from build123d import *

# Parameters (mm, degrees)
SKETCH3_W           = 186.436
SKETCH3_H           = 186.436
BOSS_EXTRUDE1_DEPTH = 3.0988
CUT_EXTRUDE1_DEPTH  = 264.678529186
CUT_EXTRUDE2_REACH  = 265.679
SKETCH5_R           = 3.175
SKETCH5_W           = 63.5
SKETCH5_H           = 63.5


with BuildPart() as part:
    # Sketch3 → Boss-Extrude1 (new body)
    with BuildSketch(Plane(origin=(0, 0, 0), x_dir=(1, 0, 0), z_dir=(0, 1, 0))):
        with Locations((93.218, 93.218)):
            Rectangle(SKETCH3_W, SKETCH3_H)
    extrude(amount=BOSS_EXTRUDE1_DEPTH)

    # Sketch4 → Cut-Extrude1 (cut, through all)
    with BuildSketch(Plane(origin=(0, 3.0988, 0), x_dir=(1, 0, 0), z_dir=(0, 1, 0))):
        with BuildLine():
            Line((5.842, 82.296), (29.718, 82.296))
            ThreePointArc((29.718, 82.296), (31.242, 80.772), (29.718, 79.248))
            Line((29.718, 79.248), (5.842, 79.248))
            ThreePointArc((5.842, 79.248), (4.318, 80.772), (5.842, 82.296))
        make_face()
        with BuildLine():
            Line((5.842, 104.14), (29.718, 104.14))
            ThreePointArc((29.718, 104.14), (31.242, 105.664), (29.718, 107.188))
            Line((29.718, 107.188), (5.842, 107.188))
            ThreePointArc((5.842, 107.188), (4.318, 105.664), (5.842, 104.14))
        make_face()
        with BuildLine():
            Line((80.772, 29.718), (80.772, 5.842))
            ThreePointArc((80.772, 5.842), (82.296, 4.318), (83.82, 5.842))
            Line((83.82, 5.842), (83.82, 29.718))
            ThreePointArc((83.82, 29.718), (82.296, 31.242), (80.772, 29.718))
        make_face()
        with BuildLine():
            Line((105.664, 5.842), (105.664, 29.718))
            ThreePointArc((105.664, 29.718), (104.14, 31.242), (102.616, 29.718))
            Line((102.616, 29.718), (102.616, 5.842))
            ThreePointArc((102.616, 5.842), (104.14, 4.318), (105.664, 5.842))
        make_face()
        with BuildLine():
            Line((156.718, 83.82), (180.594, 83.82))
            ThreePointArc((180.594, 83.82), (182.118, 82.296), (180.594, 80.772))
            Line((180.594, 80.772), (156.718, 80.772))
            ThreePointArc((156.718, 80.772), (155.194, 82.296), (156.718, 83.82))
        make_face()
        with BuildLine():
            Line((156.718, 102.616), (180.594, 102.616))
            ThreePointArc((180.594, 102.616), (182.118, 104.14), (180.594, 105.664))
            Line((180.594, 105.664), (156.718, 105.664))
            ThreePointArc((156.718, 105.664), (155.194, 104.14), (156.718, 102.616))
        make_face()
        with BuildLine():
            Line((80.772, 180.594), (80.772, 156.718))
            ThreePointArc((80.772, 156.718), (82.296, 155.194), (83.82, 156.718))
            Line((83.82, 156.718), (83.82, 180.594))
            ThreePointArc((83.82, 180.594), (82.296, 182.118), (80.772, 180.594))
        make_face()
        with BuildLine():
            Line((105.664, 156.718), (105.664, 180.594))
            ThreePointArc((105.664, 180.594), (104.14, 182.118), (102.616, 180.594))
            Line((102.616, 180.594), (102.616, 156.718))
            ThreePointArc((102.616, 156.718), (104.14, 155.194), (105.664, 156.718))
        make_face()
    extrude(amount=-CUT_EXTRUDE1_DEPTH, mode=Mode.SUBTRACT)

    # Sketch5 → Cut-Extrude2 (cut, up to next)
    with BuildSketch(Plane(origin=(0, 3.0988, 0), x_dir=(1, 0, 0), z_dir=(0, 1, 0)), mode=Mode.PRIVATE) as cut_extrude2_sk1:
        with Locations(Location((50.8, 63.5, 0), (0, 0, 270))):
            Circle(SKETCH5_R)
    cut_extrude2_tool1 = extrude(cut_extrude2_sk1.sketch, amount=-CUT_EXTRUDE2_REACH, mode=Mode.PRIVATE) & part.part
    # Sketch5 → Cut-Extrude2 (cut, up to next)
    with BuildSketch(Plane(origin=(0, 3.0988, 0), x_dir=(1, 0, 0), z_dir=(0, 1, 0)), mode=Mode.PRIVATE) as cut_extrude2_sk2:
        with Locations(Location((93.218, 63.5, 0), (0, 0, 270))):
            Circle(SKETCH5_R)
    cut_extrude2_tool2 = extrude(cut_extrude2_sk2.sketch, amount=-CUT_EXTRUDE2_REACH, mode=Mode.PRIVATE) & part.part
    # Sketch5 → Cut-Extrude2 (cut, up to next)
    with BuildSketch(Plane(origin=(0, 3.0988, 0), x_dir=(1, 0, 0), z_dir=(0, 1, 0)), mode=Mode.PRIVATE) as cut_extrude2_sk3:
        with Locations(Location((135.636, 63.5, 0), (0, 0, 270))):
            Circle(SKETCH5_R)
    cut_extrude2_tool3 = extrude(cut_extrude2_sk3.sketch, amount=-CUT_EXTRUDE2_REACH, mode=Mode.PRIVATE) & part.part
    # Sketch5 → Cut-Extrude2 (cut, up to next)
    with BuildSketch(Plane(origin=(0, 3.0988, 0), x_dir=(1, 0, 0), z_dir=(0, 1, 0)), mode=Mode.PRIVATE) as cut_extrude2_sk4:
        with Locations((93.218, 116.586)):
            Rectangle(SKETCH5_W, SKETCH5_H)
    cut_extrude2_tool4 = extrude(cut_extrude2_sk4.sketch, amount=-CUT_EXTRUDE2_REACH, mode=Mode.PRIVATE) & part.part
    add(cut_extrude2_tool1.solids().sort_by_distance((50.8, 3.0988, -63.5))[0], mode=Mode.SUBTRACT)
    add(cut_extrude2_tool2.solids().sort_by_distance((93.218, 3.0988, -63.5))[0], mode=Mode.SUBTRACT)
    add(cut_extrude2_tool3.solids().sort_by_distance((135.636, 3.0988, -63.5))[0], mode=Mode.SUBTRACT)
    add(cut_extrude2_tool4.solids().sort_by_distance((93.218, 3.0988, -116.586))[0], mode=Mode.SUBTRACT)


solid = part.part
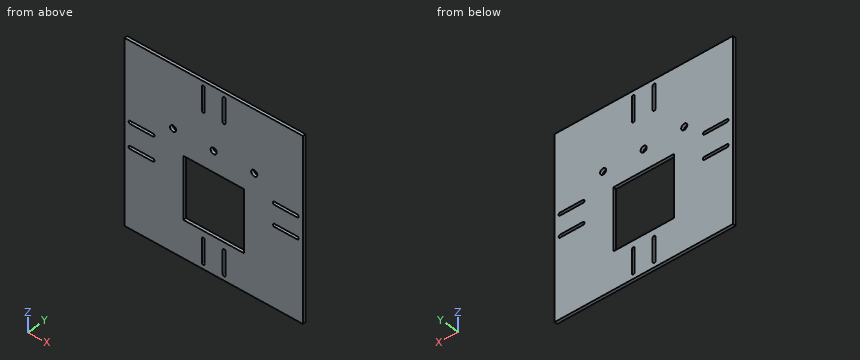
The listing builds one solid part. Answer for the finished solid, in the listing's coordinates (mm). Coordinates: 2 decimals unless noted, no trailing zeros. Loops run counter-clockwise (first coordinate to the right, second up) from the corner with the lowest first, then second, coordinate; pieces in that order, holes last. Notation, with made-up numbers: (21, 33) -> (42, 33) arc R13 cw to (42, 38) -> close; hole circle Ø8 at (67, 65.5). An arc over 180 degrees is marked (long way). Write item = value, one per line. Start each with the question number.
1) A cutting plane is placed at D-D (z = -63.5). Give the vertices of the cut face in (x, y) (3 decimals).
2) A cutting plane is placed at C-C (x = 109.5). Give the vertices of the cut face in (y, z), then the cut area to 3 significant figures.
3) A cutting plane is placed at B-B (z = -87.5). Give the vertices of the cut face in (x, y).
4) A cutting plane is placed at A-A (x = 27). Give the vertices of the cut face in (y, z), then the cut area to 3 significant figures.
5) Straight lines are drawn through the part: line 1 (X direction, y = 2.3, z = -63.5) (3 decimals); line 2 (X direction, y = 3.05, z = -20); line 3 (Z direction, x = 169, y = 2.1). For each, find the intervals that lie inside material, in ascending order. Write a range as from..to.
6) Given pin 1 Ø5.5 at (x, z) = (50.8, -63.5) entering from +Y, flat-ended and moving along its own axis, determine where the tip first touches the part or whether it passes through.
Responses:
q1.outline = (0, 0) -> (47.625, 0) -> (47.625, 3.099) -> (0, 3.099) -> close; (53.975, 0) -> (90.043, 0) -> (90.043, 3.099) -> (53.975, 3.099) -> close; (96.393, 0) -> (132.461, 0) -> (132.461, 3.099) -> (96.393, 3.099) -> close; (138.811, 0) -> (186.436, 0) -> (186.436, 3.099) -> (138.811, 3.099) -> close
q2.outline = (0, -186.44) -> (3.1, -186.44) -> (3.1, -148.34) -> (0, -148.34) -> close; (0, -84.84) -> (3.1, -84.84) -> (3.1, 0) -> (0, 0) -> close
q2.area = 381 mm²
q3.outline = (0, 0) -> (61.47, 0) -> (61.47, 3.1) -> (0, 3.1) -> close; (124.97, 0) -> (186.44, 0) -> (186.44, 3.1) -> (124.97, 3.1) -> close
q4.outline = (0, -186.44) -> (3.1, -186.44) -> (3.1, -107.19) -> (0, -107.19) -> close; (0, -104.14) -> (3.1, -104.14) -> (3.1, -82.3) -> (0, -82.3) -> close; (0, -79.25) -> (3.1, -79.25) -> (3.1, 0) -> (0, 0) -> close
q4.area = 559 mm²
q5.line_1 = 0..47.625, 53.975..90.043, 96.393..132.461, 138.811..186.436
q5.line_2 = 0..80.77, 83.82..102.62, 105.66..186.44
q5.line_3 = -186.44..-105.66, -102.62..-83.82, -80.77..0
q6.pin_1 = through
